Here's how the part is built. I have some questions about the finished solid (model axes, mm). Face numbers are marked on the shaded views. A direction names the side the tool comes from. Coordinates: 2 decimals unless noted, no trailing zeros. Loops run counter-clockwise (first coordinate to the right, second up) from the corner with the lowest first, then second, coordinate; pieces in that order, holes last. Notation, with made-up numbers: (69, 16) - (100, 16) arc R19 ccw to (100, 39) - close; hole circle Ø3 at (44, 61). An arc over 180 degrees is marked (long way). Use a Markdown table: item, result.
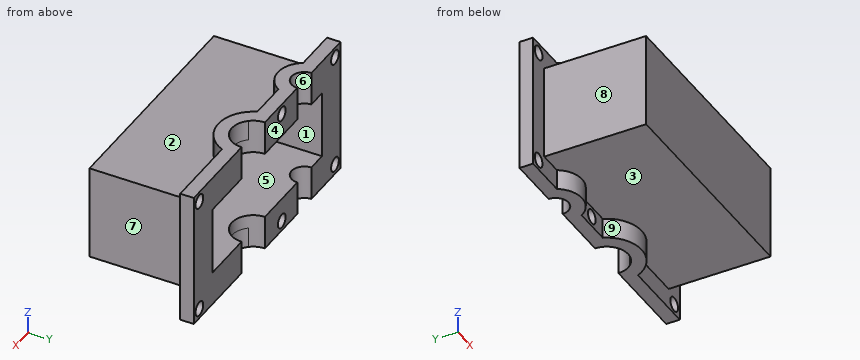
```python
from build123d import *

# Parameters (mm, degrees)
SKETCH1_W           = 42.545
SKETCH1_H           = 17.78
BOSS_EXTRUDE1_DEPTH = 2.54
SKETCH2_W           = 42.545
SKETCH2_H           = 17.78
SKETCH2_W_2         = 37.465
SKETCH2_H_2         = 12.7
EXTRUDE_THIN1_DEPTH = 19.05
SKETCH3_W           = 50.165
SKETCH3_H           = 25.4
SKETCH3_W_2         = 42.545
SKETCH3_H_2         = 17.78
BOSS_EXTRUDE2_DEPTH = 2.54
CUT_EXTRUDE1_REACH  = 43.718
SKETCH4_R           = 2.39395
SKETCH4_R_2         = 3.99415
BOSS_EXTRUDE3_START = 3.81
BOSS_EXTRUDE3_DEPTH = 3.81
BOSS_EXTRUDE4_DEPTH = 3.81
SKETCH7_R           = 1.321170669
CUT_EXTRUDE2_DEPTH  = 36.447847696


with BuildPart() as part:
    # Sketch1 → Boss-Extrude1 (new body)
    with BuildSketch(Plane(origin=(0, 0, 0), x_dir=(1, 0, 0), z_dir=(0, 1, 0))):
        Rectangle(SKETCH1_W, SKETCH1_H)
    extrude(amount=BOSS_EXTRUDE1_DEPTH)

    # Sketch2 → Extrude-Thin1 (add)
    with BuildSketch(Plane(origin=(0, 2.54, 0), x_dir=(1, 0, 0), z_dir=(0, 1, 0))):
        Rectangle(SKETCH2_W, SKETCH2_H)
        Rectangle(SKETCH2_W_2, SKETCH2_H_2, mode=Mode.SUBTRACT)
    extrude(amount=EXTRUDE_THIN1_DEPTH)

    # Sketch3 → Boss-Extrude2 (add)
    with BuildSketch(Plane(origin=(0, 21.59, 0), x_dir=(1, 0, 0), z_dir=(0, 1, 0))):
        Rectangle(SKETCH3_W, SKETCH3_H)
        Rectangle(SKETCH3_W_2, SKETCH3_H_2, mode=Mode.SUBTRACT)
    extrude(amount=-BOSS_EXTRUDE2_DEPTH)

    # Cut-Extrude1: up to this face of the body (flat: up to its plane)
    cut_extrude1_end = Plane(part.part.faces().sort_by_distance((0, 20.32, 12.7))[0])
    # Sketch4 → Cut-Extrude1 (cut, up to the picked face)
    with BuildSketch(Plane(origin=(0, 0, -12.7), x_dir=(-1, 0, 0), z_dir=(0, 0, -1)), mode=Mode.PRIVATE) as cut_extrude1_sk1:
        with Locations((12.7, 21.59)):
            Circle(SKETCH4_R)
    cut_extrude1_tool1 = split(extrude(cut_extrude1_sk1.sketch, amount=-CUT_EXTRUDE1_REACH, mode=Mode.PRIVATE), bisect_by=cut_extrude1_end, keep=Keep.BOTH, mode=Mode.PRIVATE)
    # Sketch4 → Cut-Extrude1 (cut, up to the picked face)
    with BuildSketch(Plane(origin=(0, 0, -12.7), x_dir=(-1, 0, 0), z_dir=(0, 0, -1)), mode=Mode.PRIVATE) as cut_extrude1_sk2:
        with Locations((-4.7625, 21.59)):
            Circle(SKETCH4_R_2)
    cut_extrude1_tool2 = split(extrude(cut_extrude1_sk2.sketch, amount=-CUT_EXTRUDE1_REACH, mode=Mode.PRIVATE), bisect_by=cut_extrude1_end, keep=Keep.BOTH, mode=Mode.PRIVATE)
    add(cut_extrude1_tool1.solids().sort_by(Axis((-12.7, 21.59, -12.7), (0, 0, 1)))[0], mode=Mode.SUBTRACT)
    add(cut_extrude1_tool2.solids().sort_by(Axis((4.7625, 21.59, -12.7), (0, 0, 1)))[0], mode=Mode.SUBTRACT)

    # Sketch5 → Boss-Extrude3 (add)
    with BuildSketch(Plane(origin=(0, 0, -8.89), x_dir=(-1, 0, 0), z_dir=(0, 0, -1)).offset(BOSS_EXTRUDE3_START)):
        with BuildLine():
            Line((-7.844972096, 19.05), (-10.782758817, 19.05))
            ThreePointArc((-10.782758817, 19.05), (-4.7625, 15.05585), (1.257758817, 19.05))
            Line((1.257758817, 19.05), (-1.680027904, 19.05))
            ThreePointArc((-1.680027904, 19.05), (-4.7625, 17.59585), (-7.844972096, 19.05))
        make_face()
        with BuildLine():
            Line((16.929924657, 19.05), (8.470075343, 19.05))
            ThreePointArc((8.470075343, 19.05), (12.7, 16.65605), (16.929924657, 19.05))
        make_face()
    extrude(amount=-BOSS_EXTRUDE3_DEPTH)

    # Sketch6 → Boss-Extrude4 (add)
    with BuildSketch(Plane.XY.offset(8.89)):
        with BuildLine():
            ThreePointArc((7.844972096, 19.05), (4.7625, 17.59585), (1.680027904, 19.05))
            Line((1.680027904, 19.05), (-1.257758817, 19.05))
            ThreePointArc((-1.257758817, 19.05), (4.7625, 15.05585), (10.782758817, 19.05))
            Line((10.782758817, 19.05), (7.844972096, 19.05))
        make_face()
        with BuildLine():
            ThreePointArc((-16.929924657, 19.05), (-12.7, 16.65605), (-8.470075343, 19.05))
            Line((-8.470075343, 19.05), (-16.929924657, 19.05))
        make_face()
    extrude(amount=BOSS_EXTRUDE4_DEPTH)

    # Sketch7 → Cut-Extrude2 (cut, through all)
    with BuildSketch(Plane.XZ):
        with Locations(Location((-5.000265623, 10.795, 0), (0, 0, 270))):
            Circle(SKETCH7_R)
        with Locations(Location((-5.000265623, -10.795, 0), (0, 0, 90))):
            Circle(SKETCH7_R)
        with Locations(Location((23.1775, 10.795, 0), (0, 0, 270))):
            Circle(SKETCH7_R)
        with Locations(Location((23.1775, -10.795, 0), (0, 0, 90))):
            Circle(SKETCH7_R)
        with Locations(Location((-23.1775, 10.795, 0), (0, 0, 270))):
            Circle(SKETCH7_R)
        with Locations(Location((-23.1775, -10.795, 0), (0, 0, 90))):
            Circle(SKETCH7_R)
    extrude(amount=-CUT_EXTRUDE2_DEPTH, mode=Mode.SUBTRACT)


solid = part.part
```
Q1. Which directions (+Z, -Z, +X, -X, +Y, -Y) give clear straight access to the entire face, cutting with the end or side of a thin tool? Please do the marked faces 5, 6, 7, 8 and 9.
Check values:
| item | result |
|---|---|
| face 5 | +Y |
| face 6 | +Z, -Z, +Y |
| face 7 | +Z, -Z, +X, -Y |
| face 8 | +Z, -Z, -X, -Y |
| face 9 | -Z, -Y |
Q2. Please list where these lines run through material, in increasing order: L1, parallel to Z at x = -18.5, y = 6.75; L2, parallel to X at y = 2.75, z = -4.75. Write a range as from..to.
Check values:
| item | result |
|---|---|
| L1 | -8.89..-6.35, 6.35..8.89 |
| L2 | -21.27..-18.73, 18.73..21.27 |
Q3. Will these pins go through, and if not, where does the flat tip stop? P1, Ø5.5, axis at x = -10, y = 11, coming from the +Z side; P2, Ø6.5, axis at x = 0, z = 1, coming from the +Y side; P3, Ø3, axis at x = -5, z = 10.8, coming from the -Y side.
Check values:
| item | result |
|---|---|
| P1 | z = 8.89 |
| P2 | y = 2.54 |
| P3 | y = 19.05 |
Q4. If we mould it in two halves opening along Z, with no side actions, what happens to the marked faces 1, 2, 3 and 4? For each: pulls with the +Z half, pulls with the -Z half, needs draft (parallel to the pull), parting line crosses it, or undercut.
Check values:
| item | result |
|---|---|
| face 1 | undercut |
| face 2 | pulls with the +Z half |
| face 3 | pulls with the -Z half |
| face 4 | needs draft |
Q5. I want a section at C-C, the plane z = -3.5. Write out the boundary of the cut face in (x, y), then the cut area to 3 significant figures.
Check values:
| item | result |
|---|---|
| outline | (-25.08, 19.05) - (-21.27, 19.05) - (-21.27, 0) - (21.27, 0) - (21.27, 19.05) - (25.08, 19.05) - (25.08, 21.59) - (18.73, 21.59) - (18.73, 2.54) - (-18.73, 2.54) - (-18.73, 21.59) - (-25.08, 21.59) - close |
| area | 224 mm^2 |
Q6. I want a section at A-A, the plane y = 4.5. Write out the boundary of the cut face in (x, z).
Check values:
| item | result |
|---|---|
| outline | (-21.27, -8.89) - (21.27, -8.89) - (21.27, 8.89) - (-21.27, 8.89) - close; hole (-18.73, -6.35) - (18.73, -6.35) - (18.73, 6.35) - (-18.73, 6.35) - close |
Q7. I want a section at D-D, the plane x = -4.5. Write out the boundary of the cut face in (y, z).
Check values:
| item | result |
|---|---|
| outline | (0, -8.89) - (19.05, -8.89) - (19.05, -9.57) - (21.59, -9.57) - (21.59, -6.35) - (2.54, -6.35) - (2.54, 6.35) - (21.59, 6.35) - (21.59, 9.57) - (19.05, 9.57) - (19.05, 8.89) - (0, 8.89) - close; (19.05, -12.7) - (21.59, -12.7) - (21.59, -12.02) - (19.05, -12.02) - close; (19.05, 12.02) - (21.59, 12.02) - (21.59, 12.7) - (19.05, 12.7) - close |
Q8. I want a section at B-B, the plane x = -19.5. Write out the boundary of the cut face in (y, z).
Check values:
| item | result |
|---|---|
| outline | (0, -8.89) - (19.05, -8.89) - (19.05, -12.7) - (21.59, -12.7) - (21.59, 12.7) - (19.05, 12.7) - (19.05, 8.89) - (0, 8.89) - close |
